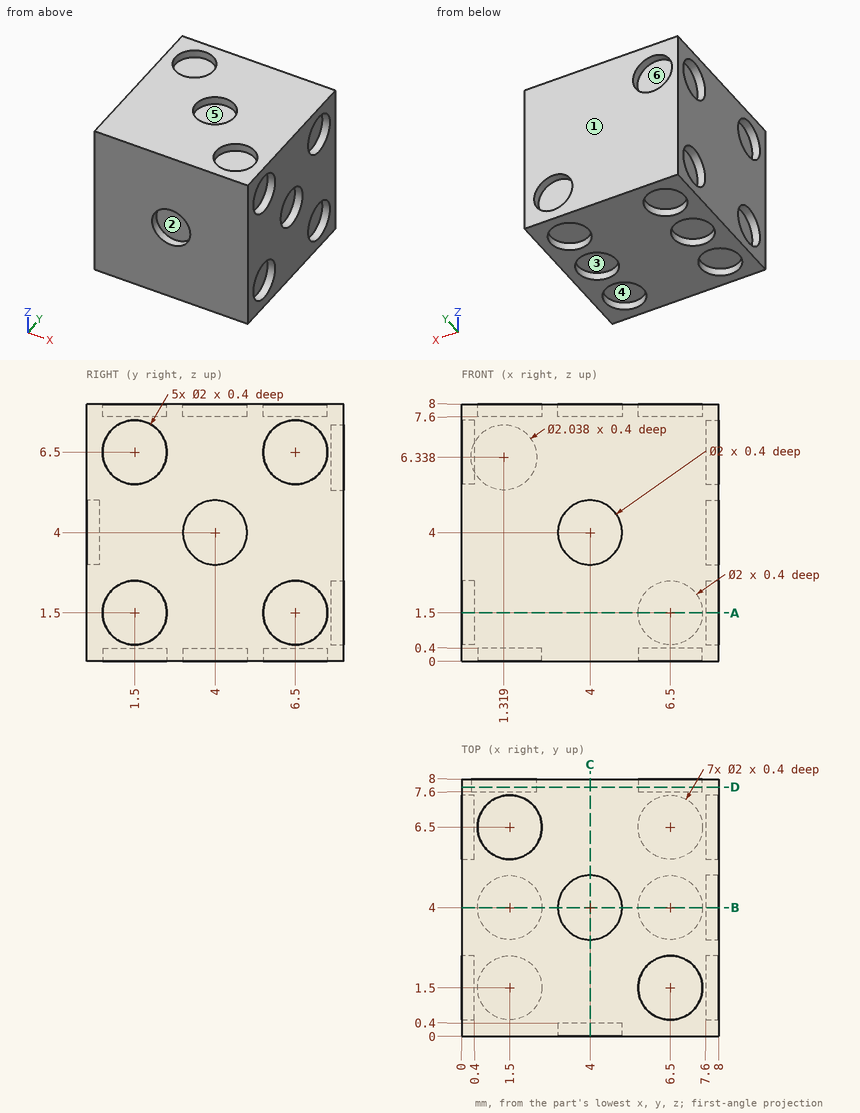
The drawing under review shows one solid part. Ordinate dimensions are in mm from its lowest x, y, z. A direction names the side the tool comes from. Coordinates: 2 decimals unless noted, no trailing zeros. Write each loop counter-clockwise with the first axis right and the second up, starting at its lowest first coordinate (ties: lowest second). Pieces come first, ordered by that corner, then holes. Notation, with made-up numbers: (88.5, 19.5) - (146.5, 19.5) arc R16 ccw to (146.5, 41.5) - close; hole circle Ø3 at (-30.5, -3.75). An arc over 180 degrees is marked (long way). Answer in a Markdown table with one row per item. Add a question column.
Q1. We need section C-C, the plane x = 4. State the section outline as (y, z) points.
Q2. Tool access review of the marked faces 4, 5 and 6: name each direction out of +Z, -Z, +X, -X, +Y, -Y from which nothing blocks a thin tool from reaching the whole face with its end or side.
Q3. For probe 1 along Y at (x, z) = (1.5, 0.35); probe 2 along X at (y, z) = (4, 0.1); probe 3 along Y at (x, z) = (1.5, 7.75), list the stretches that pass through material, from the lowest coordinate up.
Q4. We need section D-D, the plane y = 7.75. State the section outline as (x, z) points, and give its area (3 significant figures).
Q5. For P1, Ø1.8, axis at y = 6.5, z = 1.5, coming from the +X side; P2, Ø1.6, axis at x = 2, y = 6.5, coming from the -Z side; P3, Ø1.8, axis at x = 6.5, y = 1.5, coming from the +Z side; P4, Ø0.6, axis at x = 2, y = 1.5, coming from the -Z side, all flat-tipped, find the tip position at first contact; note any pin that passes through.
Q6. We need section A-A, the plane z = 1.5. State the section outline as (x, y) points.
Q7. We need section B-B, the plane y = 4. State the section outline as (x, z) points.
Q8. Draft analysis for pull direction Y (two halves, no side actions). For the marked faces 1, 2 and 3, state which applies: +Y half, -Y half, draft (parallel to the pull), parting line (faces both ways), or undercut.
Answer list:
| question | item | result |
|---|---|---|
| 1 | outline | (0, 0) - (8, 0) - (8, 8) - (5, 8) - (5, 7.6) - (3, 7.6) - (3, 8) - (0, 8) - (0, 5) - (0.4, 5) - (0.4, 3) - (0, 3) - close |
| 2 | face 4 | -Z |
| 2 | face 5 | +Z |
| 2 | face 6 | +Y |
| 3 | probe 1 | y = 0 to 0.5, 2.5 to 3, 5 to 5.5, 7.5 to 8 |
| 3 | probe 2 | x = 0 to 0.5, 2.5 to 5.5, 7.5 to 8 |
| 3 | probe 3 | y = 0 to 5.5, 7.5 to 8 |
| 4 | outline | (0, 0) - (8, 0) - (8, 8) - (0, 8) - close; hole circle Ø2.04 at (1.32, 6.34); hole circle Ø2 at (6.5, 1.5) |
| 4 | area | 57.6 mm2 |
| 5 | P1 | stops at x = 7.6 |
| 5 | P2 | stops at z = 0 |
| 5 | P3 | stops at z = 7.6 |
| 5 | P4 | stops at z = 0.4 |
| 6 | outline | (0, 0) - (8, 0) - (8, 0.5) - (7.6, 0.5) - (7.6, 2.5) - (8, 2.5) - (8, 5.5) - (7.6, 5.5) - (7.6, 7.5) - (8, 7.5) - (8, 8) - (7.5, 8) - (7.5, 7.6) - (5.5, 7.6) - (5.5, 8) - (0, 8) - (0, 7.5) - (0.4, 7.5) - (0.4, 5.5) - (0, 5.5) - (0, 2.5) - (0.4, 2.5) - (0.4, 0.5) - (0, 0.5) - close |
| 7 | outline | (0, 0) - (0.5, 0) - (0.5, 0.4) - (2.5, 0.4) - (2.5, 0) - (5.5, 0) - (5.5, 0.4) - (7.5, 0.4) - (7.5, 0) - (8, 0) - (8, 3) - (7.6, 3) - (7.6, 5) - (8, 5) - (8, 8) - (5, 8) - (5, 7.6) - (3, 7.6) - (3, 8) - (0, 8) - close |
| 8 | face 1 | +Y half |
| 8 | face 2 | -Y half |
| 8 | face 3 | undercut |
